Can you work these out from the model? Positions are in its coordinate system, mm. Face numbers are marked on the shaded views. A direction names the side the tool comes from. Round coordinates to 2 decimals unless told otherwise and drop trailing zeros. Loops run counter-clockwise (first coordinate to the right, second up) from the corner with the lowest first, then second, coordinate; pieces in that order, holes last.
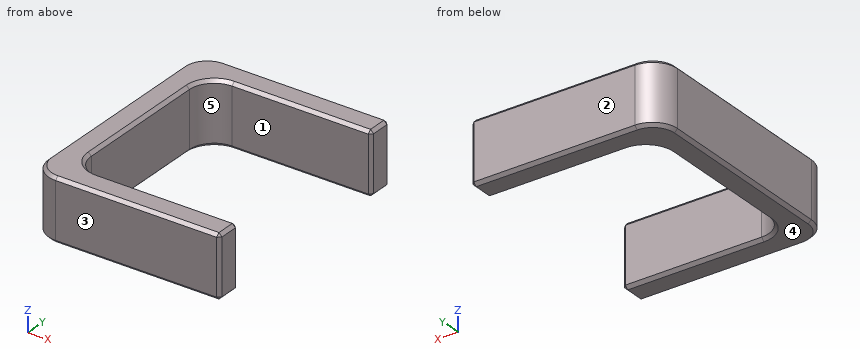
```python
from build123d import *

# Parameters (mm, degrees)
BOSS_EXTRUDE1_DEPTH = 10
FILLET1_R           = 4
CHAMFER1_SIZE       = 0.5


with BuildPart() as part:
    # Sketch1 → Boss-Extrude1 (new body)
    with BuildSketch(Plane.XY):
        Polygon((0, 0), (0, 38), (30.5, 38), (30.5, 34), (4, 34), (4, 4), (30.5, 4), (30.5, 0), align=None)
    extrude(amount=BOSS_EXTRUDE1_DEPTH)

    # Fillet1
    fillet1_edges = [part.edges().sort_by_distance(p)[0] for p in [
        (0, 0, 5),
        (0, 38, 5),
        (4, 34, 5),
        (4, 4, 5),
    ]]
    fillet(fillet1_edges, radius=FILLET1_R)

    # Chamfer1
    chamfer1_edges = [part.edges().sort_by_distance(p)[0] for p in [
        (19.25, 4, 10),
        (30.5, 2, 0),
        (30.5, 38, 5),
        (30.5, 34, 5),
        (30.5, 4, 5),
        (30.5, 0, 5),
        (30.5, 36, 10),
        (17.25, 38, 10),
        (4, 19, 0),
        (4, 19, 10),
        (19.25, 34, 0),
        (19.25, 34, 10),
        (0, 19, 0),
        (0, 19, 10),
        (17.25, 0, 0),
        (1.171572875, 1.171572875, 0),
        (1.171572875, 36.828427125, 0),
        (17.25, 0, 10),
        (1.171572875, 1.171572875, 10),
        (1.171572875, 36.828427125, 10),
        (5.171572875, 5.171572875, 0),
        (5.171572875, 5.171572875, 10),
        (5.171572875, 32.828427125, 0),
        (5.171572875, 32.828427125, 10),
        (30.5, 2, 10),
        (17.25, 38, 0),
        (30.5, 36, 0),
        (19.25, 4, 0),
    ]]
    chamfer(chamfer1_edges, length=CHAMFER1_SIZE)


solid = part.part
```
(1) We'd pull the mould along Y, two halves only. Please class the marked faces 3, 4 and 5: released by +Y, released by -Y, zero draft, split by the parting line, or undercut.
(2) Suppose I cut it at B-B (y = 14). Write out the boundary of the cut face in (x, z).
(3) Suppose I cut it at A-A (x = 24). Write out the boundary of the cut face in (y, z).
(4) Suppose I cut it at C-C (z = 8). Write out the boundary of the cut face in (x, y), then the cut area to 4 significant figures.
(5) If I drill on line 1 (Y direction, x = 17.5, z = 6.75); line 2 (X direction, y = 18, z = 5.25); line 3 (X direction, y = 2, z = 9.25), over which ranges is the centre line in solid material (lowest first)?
(6) Which directions (+Z, -Z, +X, -X, +Y, -Y) give clear straight access to the entire face, cutting with the end or side of a thin tool? Please do the marked faces 1 and 2.
Check result:
1. face 3: released by -Y
1. face 4: zero draft
1. face 5: undercut
2. outline: (0, 0.5) - (0.5, 0) - (3.5, 0) - (4, 0.5) - (4, 9.5) - (3.5, 10) - (0.5, 10) - (0, 9.5) - close
3. outline: (0, 0.5) - (0.5, 0) - (3.5, 0) - (4, 0.5) - (4, 9.5) - (3.5, 10) - (0.5, 10) - (0, 9.5) - close; (34, 0.5) - (34.5, 0) - (37.5, 0) - (38, 0.5) - (38, 9.5) - (37.5, 10) - (34.5, 10) - (34, 9.5) - close
4. outline: (0, 4) arc R4 ccw to (4, 0) - (30, 0) - (30.5, 0.5) - (30.5, 3.5) - (30, 4) - (8, 4) arc R4 cw to (4, 8) - (4, 30) arc R4 cw to (8, 34) - (30, 34) - (30.5, 34.5) - (30.5, 37.5) - (30, 38) - (4, 38) arc R4 ccw to (0, 34) - close
4. area: 363.5 mm2
5. line 1: y = 0 to 4, 34 to 38
5. line 2: x = 0 to 4
5. line 3: x = 0.54 to 30.5
6. face 1: +Z, -Z, +X
6. face 2: +Z, -Z, +X, -X, +Y
